Autodesk Fusion 360 part; units mm, degrees
sketch "Sketch1" plane through (0, 0, 0) normal (0, 0, 1) x (1, 0, 0) in component "Knob"
  circle A0 centre (0, 0) radius 3
  line L0 (-2.5981, 1.5) -> (2.5981, 1.5)
  circle A1 centre (0, 0) radius 16
  circle A2 centre (0, 16) radius 1.5
  circle A3 centre (-8, 13.8564) radius 1.5
  circle A4 centre (-13.8564, 8) radius 1.5
  circle A5 centre (-16, 0) radius 1.5
  circle A6 centre (-13.8564, -8) radius 1.5
  circle A7 centre (-8, -13.8564) radius 1.5
  circle A8 centre (0, -16) radius 1.5
  circle A9 centre (8, -13.8564) radius 1.5
  circle A10 centre (13.8564, -8) radius 1.5
  circle A11 centre (16, 0) radius 1.5
  circle A12 centre (13.8564, 8) radius 1.5
  circle A13 centre (8, 13.8564) radius 1.5
  point P0 (0, -3)
  dimension "d1" = 6
  dimension "d3" = 4.5
  dimension "d4" = 32
  dimension "d5" = 3
  dimension "d7" = 360
extrude "Extrude1" add sketch "Sketch1" along normal blind 12 contours A0 L0 | A1 A11 | A1 A11 | A1 A2 A3 A4 A5 A6 A7 A8 A9 A10 A11 A12 A13 | A1 A12 | A1 A12 | A1 A10 | A1 A10 | A1 A13 | A1 A13 | A1 A9 | A1 A9 | A1 A2 | A1 A2 | A1 A8 | A1 A8 | A1 A3 | A1 A3 | A1 A7 | A1 A7 | A1 A4 | A1 A4 | A1 A6 | A1 A6 | A1 A5 | A1 A5 picked at (0.8914, -0.3917) in component "Knob"
extrude "Extrude2" add sketch "Sketch1" along normal blind 3 from surface at 12 contours A0 L0 | A0 L0 | A1 A11 | A1 A11 | A1 A2 A3 A4 A5 A6 A7 A8 A9 A10 A11 A12 A13 | A1 A12 | A1 A12 | A1 A10 | A1 A10 | A1 A13 | A1 A13 | A1 A9 | A1 A9 | A1 A2 | A1 A2 | A1 A8 | A1 A8 | A1 A3 | A1 A3 | A1 A7 | A1 A7 | A1 A4 | A1 A4 | A1 A6 | A1 A6 | A1 A5 | A1 A5 in component "Knob"
sketch "Sketch2" plane through (0, 0, 15) normal (0, 0, 1) x (-1, 0, 0) in component "Knob"
  arc A0 (-9.2625, -13.0463) -> (-6.6672, -14.5447) centre (-8, -13.8564) ccw
  arc A1 (-6.6672, -14.5447) -> (-1.4984, -15.9297) centre (0, 0) ccw
  arc A2 (-1.4984, -15.9297) -> (1.4984, -15.9297) centre (0, -16) ccw
  arc A3 (1.4984, -15.9297) -> (6.6672, -14.5447) centre (0, 0) ccw
  arc A4 (6.6672, -14.5447) -> (9.2625, -13.0463) centre (8, -13.8564) ccw
  arc A5 (9.2625, -13.0463) -> (13.0463, -9.2625) centre (0, 0) ccw
  arc A6 (13.0463, -9.2625) -> (14.5447, -6.6672) centre (13.8564, -8) ccw
  arc A7 (14.5447, -6.6672) -> (15.9297, -1.4984) centre (0, 0) ccw
  arc A8 (15.9297, -1.4984) -> (15.9297, 1.4984) centre (16, 0) ccw
  arc A9 (15.9297, 1.4984) -> (14.5447, 6.6672) centre (0, 0) ccw
  arc A10 (14.5447, 6.6672) -> (13.0463, 9.2625) centre (13.8564, 8) ccw
  arc A11 (13.0463, 9.2625) -> (9.2625, 13.0463) centre (0, 0) ccw
  arc A12 (9.2625, 13.0463) -> (6.6672, 14.5447) centre (8, 13.8564) ccw
  arc A13 (6.6672, 14.5447) -> (1.4984, 15.9297) centre (0, 0) ccw
  arc A14 (1.4984, 15.9297) -> (-1.4984, 15.9297) centre (0, 16) ccw
  arc A15 (-1.4984, 15.9297) -> (-6.6672, 14.5447) centre (0, 0) ccw
  arc A16 (-6.6672, 14.5447) -> (-9.2625, 13.0463) centre (-8, 13.8564) ccw
  arc A17 (-9.2625, 13.0463) -> (-13.0463, 9.2625) centre (0, 0) ccw
  arc A18 (-13.0463, 9.2625) -> (-14.5447, 6.6672) centre (-13.8564, 8) ccw
  arc A19 (-14.5447, 6.6672) -> (-15.9297, 1.4984) centre (0, 0) ccw
  arc A20 (-15.9297, 1.4984) -> (-15.9297, -1.4984) centre (-16, 0) ccw
  arc A21 (-15.9297, -1.4984) -> (-14.5447, -6.6672) centre (0, 0) ccw
  arc A22 (-14.5447, -6.6672) -> (-13.0463, -9.2625) centre (-13.8564, -8) ccw
  arc A23 (-13.0463, -9.2625) -> (-9.2625, -13.0463) centre (0, 0) ccw
  line L0 (0.5, -15) -> (-0.5, -15)
  line L1 (-0.5, -15) -> (-0.5, -4)
  line L2 (-0.5, -4) -> (0.5, -4)
  line L3 (0.5, -4) -> (0.5, -15)
  line L4 (1.567, -3.7141) -> (2.433, -3.2141)
  line L5 (2.433, -3.2141) -> (7.933, -12.7404)
  line L6 (7.067, -13.2404) -> (1.567, -3.7141)
  line L7 (7.933, -12.7404) -> (7.067, -13.2404)
  line L8 (3.2141, -2.433) -> (3.7141, -1.567)
  line L9 (3.7141, -1.567) -> (13.2404, -7.067)
  line L10 (12.7404, -7.933) -> (3.2141, -2.433)
  line L11 (13.2404, -7.067) -> (12.7404, -7.933)
  line L12 (4, -0.5) -> (4, 0.5)
  line L13 (4, 0.5) -> (15, 0.5)
  line L14 (15, -0.5) -> (4, -0.5)
  line L15 (15, 0.5) -> (15, -0.5)
  line L16 (3.7141, 1.567) -> (3.2141, 2.433)
  line L17 (3.2141, 2.433) -> (12.7404, 7.933)
  line L18 (13.2404, 7.067) -> (3.7141, 1.567)
  line L19 (12.7404, 7.933) -> (13.2404, 7.067)
  line L20 (2.433, 3.2141) -> (1.567, 3.7141)
  line L21 (1.567, 3.7141) -> (7.067, 13.2404)
  line L22 (7.933, 12.7404) -> (2.433, 3.2141)
  line L23 (7.067, 13.2404) -> (7.933, 12.7404)
  line L24 (0.5, 4) -> (-0.5, 4)
  line L25 (-0.5, 4) -> (-0.5, 15)
  line L26 (0.5, 15) -> (0.5, 4)
  line L27 (-0.5, 15) -> (0.5, 15)
  line L28 (-1.567, 3.7141) -> (-2.433, 3.2141)
  line L29 (-2.433, 3.2141) -> (-7.933, 12.7404)
  line L30 (-7.067, 13.2404) -> (-1.567, 3.7141)
  line L31 (-7.933, 12.7404) -> (-7.067, 13.2404)
  line L32 (-3.2141, 2.433) -> (-3.7141, 1.567)
  line L33 (-3.7141, 1.567) -> (-13.2404, 7.067)
  line L34 (-12.7404, 7.933) -> (-3.2141, 2.433)
  line L35 (-13.2404, 7.067) -> (-12.7404, 7.933)
  line L36 (-4, 0.5) -> (-4, -0.5)
  line L37 (-4, -0.5) -> (-15, -0.5)
  line L38 (-15, 0.5) -> (-4, 0.5)
  line L39 (-15, -0.5) -> (-15, 0.5)
  line L40 (-3.7141, -1.567) -> (-3.2141, -2.433)
  line L41 (-3.2141, -2.433) -> (-12.7404, -7.933)
  line L42 (-13.2404, -7.067) -> (-3.7141, -1.567)
  line L43 (-12.7404, -7.933) -> (-13.2404, -7.067)
  line L44 (-2.433, -3.2141) -> (-1.567, -3.7141)
  line L45 (-1.567, -3.7141) -> (-7.067, -13.2404)
  line L46 (-7.933, -12.7404) -> (-2.433, -3.2141)
  line L47 (-7.067, -13.2404) -> (-7.933, -12.7404)
  dimension "d18" = 11
  dimension "d19" = 1
  dimension "d20" = 0.5
  dimension "d21" = 4
  dimension "d23" = 360
component "Knob" placed x (1, 0, 0) y (0, 1, 0) z (0, 0, 1) at (0, 0, 0)
equation "d20 = d19 / 2"
Source: CAD feature listing. Evaluate the final solid. Frame: model axes, mm. A direction names the side the tool comes from. Coordinates: 2 decimals unless noted, no trailing zeros. Write each loop counter-clockwise with the first axis right and the second up, starting at its lowest first coordinate (ties: lowest second). Pieces come first, ordered by that corner, then holes. Notation, with made-up numbers: M -8.75,-26.75 L 2.25,-26.75 A10 cw 2.25,-11.75 Z; hole C -22.5,69.5 d9. An arc over 180 degrees is marked long. Answer as a JSON object with one key per item and string values.
1. Cut plane C-C on x = 0. Output: boundary loops of the cut face in (y, z), plus the area to 3 significant figures.
Evaluation:
{"outline": "M -17.5,0 L 1.5,0 L 1.5,12 L 3,12 L 3,0 L 17.5,0 L 17.5,15 L -17.5,15 Z", "area": "507 mm^2"}
2. Draft query along X for faces 1 (the cylindrical face through (15.465, -4.105, 7.395)), 2 (the flat face through (0, 0, 15)), 3 (the cylindrical face through (15.172, -8.72, 7.395)). Return one class per face: released by +X, released by -X, zero draft, split by the parting line, or undercut.
Evaluation:
{"face 1": "released by +X", "face 2": "zero draft", "face 3": "undercut"}
3. Access query for faces 4 (the cylindrical face through (4.177, -15.445, 7.395)), 5 (the flat face through (0, 2, 12)), 6 (the cylindrical face through (4.105, 15.465, 7.395)), 7 (the cylindrical face through (-15.445, -4.177, 7.395)). Directions: +Z, -Z, +X, -X, +Y, -Y. A direction counts if a zero-diameter tool reaches every point of the face in a straight line with its end or side. Return the directions, or none.
Evaluation:
{"face 4": "+Z, -Z, -Y", "face 5": "-Z", "face 6": "+Z, -Z, +Y", "face 7": "+Z, -Z, -X"}
4. Cut plane A-A on z = 9.5. Output: boundary loops of the cut face in (x, y).
Evaluation:
{"outline": "M -15.93,-1.5 A16 ccw -14.54,-6.67 A1.5 ccw long -13.05,-9.26 A16 ccw -9.26,-13.05 A1.5 ccw long -6.67,-14.54 A16 ccw -1.5,-15.93 A1.5 ccw long 1.5,-15.93 A16 ccw 6.67,-14.54 A1.5 ccw long 9.26,-13.05 A16 ccw 13.05,-9.26 A1.5 ccw long 14.54,-6.67 A16 ccw 15.93,-1.5 A1.5 ccw long 15.93,1.5 A16 ccw 14.54,6.67 A1.5 ccw long 13.05,9.26 A16 ccw 9.26,13.05 A1.5 ccw long 6.67,14.54 A16 ccw 1.5,15.93 A1.5 ccw long -1.5,15.93 A16 ccw -6.67,14.54 A1.5 ccw long -9.26,13.05 A16 ccw -13.05,9.26 A1.5 ccw long -14.54,6.67 A16 ccw -15.93,1.5 A1.5 ccw long Z; hole M -2.6,1.5 L 2.6,1.5 A3 ccw Z"}
5. Cut plane D-D on y = 10. Output: boundary loops of the cut face in (x, z), plus the area to 3 significant figures.
Evaluation:
{"outline": "M -12.49,0 L 12.49,0 L 12.49,15 L -12.49,15 Z", "area": "375 mm^2"}
6. Cut plane B-B on z = 13. Output: boundary loops of the cut face in (x, y).
Evaluation:
{"outline": "M -15.93,-1.5 A16 ccw -14.54,-6.67 A1.5 ccw long -13.05,-9.26 A16 ccw -9.26,-13.05 A1.5 ccw long -6.67,-14.54 A16 ccw -1.5,-15.93 A1.5 ccw long 1.5,-15.93 A16 ccw 6.67,-14.54 A1.5 ccw long 9.26,-13.05 A16 ccw 13.05,-9.26 A1.5 ccw long 14.54,-6.67 A16 ccw 15.93,-1.5 A1.5 ccw long 15.93,1.5 A16 ccw 14.54,6.67 A1.5 ccw long 13.05,9.26 A16 ccw 9.26,13.05 A1.5 ccw long 6.67,14.54 A16 ccw 1.5,15.93 A1.5 ccw long -1.5,15.93 A16 ccw -6.67,14.54 A1.5 ccw long -9.26,13.05 A16 ccw -13.05,9.26 A1.5 ccw long -14.54,6.67 A16 ccw -15.93,1.5 A1.5 ccw long Z"}
7. Contact query for flat-ended pins moving along their axis: P1, Ø6, axis at x = 4, z = 2.5, coming from the +Y side; P2, Ø3, axis at y = -4, z = 6.5, coming from the -X side; P3, Ø3, axis at y = 11.5, z = 4, coming from the -X side. Output: stop coordinate, or through.
Evaluation:
{"P1": "y = 17.12", "P2": "x = -15.8", "P3": "x = -12.49"}
8. Ray query, L1, parallel to Z at x = 1.5, y = 2.5; L2, parallel to Y at x = -16, z = 11.5; L3, parallel to Y at x = -2, z = 6.75. Return the intervals inside material, ascending.
Evaluation:
{"L1": "12 to 15", "L2": "-1.5 to 1.5", "L3": "-15.87 to 1.5, 2.24 to 15.87"}
